from build123d import *

# Parameters (mm, degrees)
SKETCH1_R           = 1.55
SKETCH1_W           = 354.775
SKETCH1_H           = 97.6
BOSS_EXTRUDE1_DEPTH = 3


with BuildPart() as part:
    # Sketch1 → Boss-Extrude1 (new body)
    with BuildSketch(Plane(origin=(0, 0, 0), x_dir=(1, 0, 0), z_dir=(0, 1, 0))):
        with BuildLine():
            Line((-2.165e-06, 108.600001782), (-2.165e-06, 5.000001782))
            ThreePointArc((-2.165e-06, 5.000001782), (1.464463929, 1.464467876), (4.999997835, 1.782e-06))
            Line((4.999997835, 1.782e-06), (365.774997835, 1.782e-06))
            ThreePointArc((365.774997835, 1.782e-06), (369.31053174, 1.464467876), (370.774997835, 5.000001782))
            Line((370.774997835, 5.000001782), (370.774997835, 108.600001782))
            ThreePointArc((370.774997835, 108.600001782), (369.31053174, 112.135535688), (365.774997835, 113.600001782))
            Line((365.774997835, 113.600001782), (4.999997835, 113.600001782))
            ThreePointArc((4.999997835, 113.600001782), (1.464463929, 112.135535688), (-2.165e-06, 108.600001782))
        make_face()
        with Locations(Location((195.387497835, 109.100001782, 0), (0, 0, 270))):
            Circle(SKETCH1_R, mode=Mode.SUBTRACT)
        with Locations(Location((175.387497835, 109.100001782, 0), (0, 0, 270))):
            Circle(SKETCH1_R, mode=Mode.SUBTRACT)
        with Locations(Location((85.387497835, 107.600001782, 0), (0, 0, 270))):
            Circle(SKETCH1_R, mode=Mode.SUBTRACT)
        with Locations(Location((285.387497835, 107.600001782, 0), (0, 0, 270))):
            Circle(SKETCH1_R, mode=Mode.SUBTRACT)
        with Locations(Location((85.387497835, 6.000001782, 0), (0, 0, 270))):
            Circle(SKETCH1_R, mode=Mode.SUBTRACT)
        with Locations(Location((185.387497835, 6.000001782, 0), (0, 0, 270))):
            Circle(SKETCH1_R, mode=Mode.SUBTRACT)
        with Locations(Location((285.387497835, 6.000001782, 0), (0, 0, 270))):
            Circle(SKETCH1_R, mode=Mode.SUBTRACT)
        with Locations((185.387497835, 56.800001782)):
            Rectangle(SKETCH1_W, SKETCH1_H, mode=Mode.SUBTRACT)
        Polygon((234.088459729, 111.350001782), (236.68653594, 111.350001782), (237.985574046, 109.100001782), (236.68653594, 106.850001782), (234.088459729, 106.850001782), (232.789421623, 109.100001782), align=None, mode=Mode.SUBTRACT)
        Polygon((334.088459729, 111.350001782), (336.68653594, 111.350001782), (337.985574046, 109.100001782), (336.68653594, 106.850001782), (334.088459729, 106.850001782), (332.789421623, 109.100001782), align=None, mode=Mode.SUBTRACT)
        Polygon((365.947429439, 110.609550693), (367.784546746, 108.772433386), (367.112115142, 106.262884475), (364.60256623, 105.590452871), (362.765448923, 107.427570178), (363.437880527, 109.937119089), align=None, mode=Mode.SUBTRACT)
        Polygon((136.68653594, 111.350001782), (134.088459729, 111.350001782), (132.789421623, 109.100001782), (134.088459729, 106.850001782), (136.68653594, 106.850001782), (137.985574046, 109.100001782), align=None, mode=Mode.SUBTRACT)
        Polygon((36.68653594, 111.350001782), (34.088459729, 111.350001782), (32.789421623, 109.100001782), (34.088459729, 106.850001782), (36.68653594, 106.850001782), (37.985574046, 109.100001782), align=None, mode=Mode.SUBTRACT)
        Polygon((4.82756623, 110.609550693), (2.990448923, 108.772433386), (3.662880527, 106.262884475), (6.172429439, 105.590452871), (8.009546746, 107.427570178), (7.337115142, 109.937119089), align=None, mode=Mode.SUBTRACT)
        Polygon((234.088459729, 2.250001782), (236.68653594, 2.250001782), (237.985574046, 4.500001782), (236.68653594, 6.750001782), (234.088459729, 6.750001782), (232.789421623, 4.500001782), align=None, mode=Mode.SUBTRACT)
        Polygon((334.088459729, 2.250001782), (336.68653594, 2.250001782), (337.985574046, 4.500001782), (336.68653594, 6.750001782), (334.088459729, 6.750001782), (332.789421623, 4.500001782), align=None, mode=Mode.SUBTRACT)
        Polygon((365.947429439, 2.990452871), (367.784546746, 4.827570178), (367.112115142, 7.337119089), (364.60256623, 8.009550693), (362.765448923, 6.172433386), (363.437880527, 3.662884475), align=None, mode=Mode.SUBTRACT)
        Polygon((136.68653594, 2.250001782), (134.088459729, 2.250001782), (132.789421623, 4.500001782), (134.088459729, 6.750001782), (136.68653594, 6.750001782), (137.985574046, 4.500001782), align=None, mode=Mode.SUBTRACT)
        Polygon((36.68653594, 2.250001782), (34.088459729, 2.250001782), (32.789421623, 4.500001782), (34.088459729, 6.750001782), (36.68653594, 6.750001782), (37.985574046, 4.500001782), align=None, mode=Mode.SUBTRACT)
        Polygon((4.82756623, 2.990452871), (2.990448923, 4.827570178), (3.662880527, 7.337119089), (6.172429439, 8.009550693), (8.009546746, 6.172433386), (7.337115142, 3.662884475), align=None, mode=Mode.SUBTRACT)
    extrude(amount=-BOSS_EXTRUDE1_DEPTH)


solid = part.part
Could you check a few things on this model? Use its own coordinates, in mm. Coordinates: 2 decimals unless noted, no trailing zeros. Order: outer loops, then holes, each group sorted by start corner. A loop starts at its lowest first (then second) coordinate and runs counter-clockwise, first axis right, second up. Notation, with made-up numbers: (-1.5, 70) -> (49.5, 70) arc R16 ccw to (49.5, 100) -> close; hole circle Ø11 at (36, -22). An arc over 180 degrees is marked (long way). One line per question, with ' | ' between items.
Q1. Imagine slicing it at C-C on y = -1.85. State how many separate pieces and enclosed holes the cut face has, and give its area (3 significant figures).
Return value:
separate pieces: 1 | enclosed holes: 20 | area: 7,210 mm²
Q2. If I drill on L1, parallel to X at y = -1.9, z = -55 (3 decimals); L2, parallel to Z at x = 279, y = -2.25, over which ranges is the centre line in solid material (lowest first)?
Return value:
L1: 0 to 8, 362.775 to 370.775 | L2: -113.6 to -105.6, -8 to 0
Q3. Imagine slicing it at B-B on x = 91. Please give me the cut outline in (y, z).
Return value:
outline: (-3, -113.6) -> (0, -113.6) -> (0, -105.6) -> (-3, -105.6) -> close; (-3, -8) -> (0, -8) -> (0, 0) -> (-3, 0) -> close
Q4. Imagine slicing it at A-A on z = -84. Please give me the cut outline in (x, y) (3 decimals).
Return value:
outline: (0, -3) -> (8, -3) -> (8, 0) -> (0, 0) -> close; (362.775, -3) -> (370.775, -3) -> (370.775, 0) -> (362.775, 0) -> close
